```python
from build123d import *

# Parameters (mm, degrees)
SKETCH_1_W             = 35
SKETCH_1_H             = 37
EXTRUDE_1_DEPTH        = 0.1
EXTRUDE_2_DEPTH        = 0.1
EXTRUDE_3_DEPTH        = 0.1
PATTERN_LINEAR_1_COUNT = 2
PATTERN_LINEAR_1_PITCH = 36.9
PATTERN_LINEAR_2_COUNT = 2
PATTERN_LINEAR_2_PITCH = 34.9


with BuildPart() as part:
    # 草图1 → 凸台-拉伸1 (new body)
    with BuildSketch(Plane(origin=(0, 0, 0), x_dir=(1, 0, 0), z_dir=(0, 1, 0))):
        with Locations((17.5, 18.5)):
            Rectangle(SKETCH_1_W, SKETCH_1_H)
    extrude(amount=-EXTRUDE_1_DEPTH)

    # 草图2 → 拉伸-薄壁2 (add)
    with BuildSketch(Plane.XY):
        Polygon((0, 0), (0, 1.8), (6, 1.8), (6, 0.8), (7.5, 0.8), (7.5, 1.8), (27.5, 1.8), (27.5, 0.8), (29, 0.8), (29, 1.8), (35, 1.8), (35, 0), (34.9, 0), (34.9, 1.7), (29.1, 1.7), (29.1, 0.7), (27.4, 0.7), (27.4, 1.7), (7.6, 1.7), (7.6, 0.7), (5.9, 0.7), (5.9, 1.7), (0.1, 1.7), (0.1, 0), align=None)
    extrude_2 = extrude(amount=-EXTRUDE_2_DEPTH)

    # 草图3 → 拉伸-薄壁3 (add)
    with BuildSketch(Plane(origin=(0, 0, 0), x_dir=(0, 0, -1), z_dir=(1, 0, 0))):
        Polygon((0, 1.8), (6.5, 1.8), (6.5, 0.8), (8, 0.8), (8, 1.8), (29, 1.8), (29, 0.8), (30.5, 0.8), (30.5, 1.8), (37, 1.8), (37, 0), (36.9, 0), (36.9, 1.7), (30.6, 1.7), (30.6, 0.7), (28.9, 0.7), (28.9, 1.7), (8.1, 1.7), (8.1, 0.7), (6.4, 0.7), (6.4, 1.7), (0, 1.7), align=None)
    extrude_3 = extrude(amount=EXTRUDE_3_DEPTH)

    # 阵列(线性)1: 拉伸-薄壁2 ×2
    with Locations(*[(0, 0, -i * PATTERN_LINEAR_1_PITCH) for i in range(1, PATTERN_LINEAR_1_COUNT)]):
        add(extrude_2)

    # 阵列(线性)2: 拉伸-薄壁3 ×2
    with Locations(*[(i * PATTERN_LINEAR_2_PITCH, 0, 0) for i in range(1, PATTERN_LINEAR_2_COUNT)]):
        add(extrude_3)


solid = part.part
```
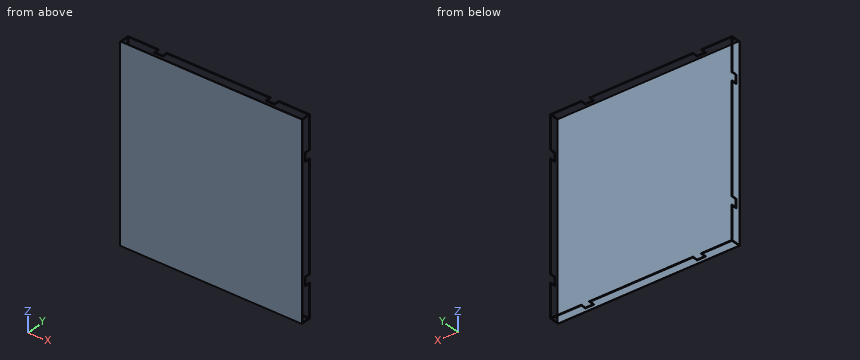
Source: CAD feature listing. Evaluate the final solid. Frame: model axes, mm. Round coordinates to 2 decimals unless told otherwise and drop trailing zeros. Loops run counter-clockwise (first coordinate to the right, second up) from the corner with the lowest first, then second, coordinate; pieces in that order, holes last. Notation, with made-up numbers: M 23,-8 L 47,-8 A21 ccw 47,12 Z; hole C 7.25,12 d11. An arc over 180 degrees is marked long. Use a Markdown table: item, result. Add a question column.
1. Section query B-B on x = 25.5. Return the cut outline in (y, z), then the cut area to 3 significant figures.
2. Section query A-A on z = -24.5. Return the cut outline in (x, y), then the cut area to 3 significant figures.
3. Contact query for a flat-ended pin moving along its axis: P1, Ø5, axis at x = 15.5, z = -29, coming from the +Y side. Output: stop coordinate, or through.
4. Section query C-C on y = 1.2. Give the number of separate pieces and of enclosed holes in the cut face, then the cut area to 3 significant figures.
Reported:
| question | item | result |
|---|---|---|
| 1 | outline | M -0.1,-37 L 0,-37 L 0,0 L -0.1,0 Z; M 1.7,-37 L 1.8,-37 L 1.8,-36.9 L 1.7,-36.9 Z; M 1.7,-0.1 L 1.8,-0.1 L 1.8,0 L 1.7,0 Z |
| 1 | area | 3.72 mm² |
| 2 | outline | M 0,-0.1 L 35,-0.1 L 35,0 L 0,0 Z; M 0,1.7 L 0.1,1.7 L 0.1,1.8 L 0,1.8 Z; M 34.9,1.7 L 35,1.7 L 35,1.8 L 34.9,1.8 Z |
| 2 | area | 3.52 mm² |
| 3 | P1 | stops at y = 0 |
| 4 | separate pieces | 20 |
| 4 | enclosed holes | 0 |
| 4 | area | 0.200 mm² |
